```python
from build123d import *

# Parameters (mm, degrees)
F1_DEPTH = 76.2
F3_DEPTH = 59.69


with BuildPart() as f1:
    # F0 (on Front) → F1 (new body)
    with BuildSketch(Plane.XZ):
        Polygon((-9.623217, -31.607002), (0, -26.720898), (9.005067, -12.367957), (23.358002, -30.080097), (23.968766, -5.954943), (42.902432, -17.254066), (29.160259, 4.122653), (48.704684, 14.200249), (23.968766, 14.200249), (31.908695, 39.85231), (12.975028, 16.643301), (12.975028, 45.043796), (5.340484, 18.780973), (0, 43.822274), (-7.790928, 17.559446), (-21.227721, 42.295363), (-13.287797, 13.284104), (-29.167645, 19.086355), (-16.952377, 8.703378), (-36.70152, -2.024551), (-17.56314, -11.757195), (-35.789758, -21.658073), (-9.623217, -15.727157), align=None)
    extrude(amount=F1_DEPTH)

    # F2 (on face) → F3 (cut)
    with BuildSketch(Plane.XZ.offset(76.2)):
        Polygon((21.212701, 12.168249), (26.877798, 30.47086), (10.943028, 10.937917), (10.943028, 30.774279), (5.037519, 10.459334), (-0.322264, 35.591124), (-7.236843, 12.282424), (-14.633635, 25.899247), (-10.289114, 10.025038), (-19.200415, 13.281089), (-13.378382, 8.332362), (-32.335366, -1.965259), (-13.196986, -11.697903), (-21.902551, -16.426851), (-7.591217, -13.18304), (-7.591217, -28.296349), (-1.422014, -25.16399), (8.794351, -8.880393), (21.466165, -24.517956), (22.025383, -2.428849), (36.515134, -11.075958), (26.24216, 4.904228), (40.329954, 12.168249), align=None)
    extrude(amount=-F3_DEPTH, mode=Mode.SUBTRACT)


solid = f1.part
```
The model under review builds one solid part; all positions refer to its coordinate system, in mm. A direction names the side the tool comes from. Give positions to 0.01 mm unless a question says otherwise; leave off trailing zeros. Order: outer loops, then holes, each group sorted by start corner. A loop starts at its lowest first (then second) coordinate and runs counter-clockwise, first axis right, second up. Notation, with made-up numbers: (2.5, 45) - (9.5, 45) arc R12 cw to (9.5, 60) - close; hole circle Ø1 at (-17, 31.25). An arc over 180 degrees is marked (long way). Use CSV: the item, a comma, the result in double quotes. Start each with the question number.
Q1. Tool access review of faces 1 (the flat face through (16, -38, -21)), 2 (the flat face through (36.13, -37.57, -6.72)), 3 (the flat face through (-26.689, -37.567, 3.415)), 4 (the flat face through (22.574, -37.567, 28.41)), 5 (the flat face through (-22.72, -46.77, 3.26)): name each direction out of +Z, -Z, +X, -X, +Y, -Y from which nothing blocks a thin tool from reaching the whole face with its end or side.
Q2. We need section D-D, the plane x = 38.5. Write out the cut boundary in (y, z).
Q3. To check wall thickness, follow line 1 along X through (y, z) = (-13.5, -13.5); line 2 along X through (y, z) = (-5, 37); line 3 along Z through (x, y) = (33.5, -30). State the ranges of each line that lie inside material, in increasing order. Write a range as [from, to].
Q4. The part is to be moulded in two halves that separate along X. For faces 6 (the flat face through (5, 0, -1)), 7 (the flat face through (-14.85, -46.77, -14.83)), 8 (the flat face through (38.796, -37.567, 9.091)), say which applies: +X half, -X half, draft (parallel to the pull), parting line (faces both ways), or undercut.
Q5. We need section C-C, the plane y = -13. Write out the cut boundary in (x, z), and give its area (3 significant figures).
Q6. We need section B-B, the plane x = -25.5. Write out the cut boundary in (y, z), and give its area (3 significant figures).
Q7. We need section A-A, the plane z = -19.5. Write out the cut boundary in (x, y).
Q8. Clearance check with flat-ended pins moving along their axes: pin 1 Ø1.5 at (y, z) = (-62, -15.5) entering from +X; pin 2 Ø2 at (x, z) = (-1, 26.5) entering from +Y; pin 3 Ø8 at (y, z) = (-56.5, -3) entering from -X; pin 4 Ø1.5 at (x, z) = (3, -6) entering from -Y. State where each tip first meets the part, or that it passes through.
Outcome:
1,face 1,"-Z, +Y, -Y"
1,face 2,"+X, +Y, -Y"
1,face 3,"-X, +Y, -Y"
1,face 4,"+Z, +Y, -Y"
1,face 5,"-Y"
2,outline,"(-76.2, -14.63) - (0, -14.63) - (0, -10.41) - (-76.2, -10.41) - close; (-76.2, 8.94) - (0, 8.94) - (0, 14.2) - (-76.2, 14.2) - (-76.2, 12.17) - (-16.51, 12.17) - (-16.51, 11.22) - (-76.2, 11.22) - close"
3,line 1,"x = [-20.77, 8.29], [9.92, 23.78], [36.61, 40.49]"
3,line 2,"x = [-19.78, -18.35], [-2.02, 1.45], [10.64, 12.98], [29.58, 31.03]"
3,line 3,"z = [-11.64, -9.28], [-6.39, -2.63], [6.36, 8.65], [12.17, 14.2]"
4,face 6,"draft"
4,face 7,"undercut"
4,face 8,"+X half"
5,outline,"(-36.7, -2.02) - (-17.56, -11.76) - (-35.79, -21.66) - (-9.62, -15.73) - (-9.62, -31.61) - (0, -26.72) - (9.01, -12.37) - (23.36, -30.08) - (23.97, -5.95) - (42.9, -17.25) - (29.16, 4.12) - (48.7, 14.2) - (23.97, 14.2) - (31.91, 39.85) - (12.98, 16.64) - (12.98, 45.04) - (5.34, 18.78) - (0, 43.82) - (-7.79, 17.56) - (-21.23, 42.3) - (-13.29, 13.28) - (-29.17, 19.09) - (-16.95, 8.7) - close"
5,area,"2,700 mm^2"
6,outline,"(-76.2, -19.33) - (0, -19.33) - (0, -16.07) - (-76.2, -16.07) - close; (-76.2, -7.72) - (0, -7.72) - (0, 4.06) - (-76.2, 4.06) - (-76.2, 1.75) - (-16.51, 1.75) - (-16.51, -5.44) - (-76.2, -5.44) - close; (-76.2, 15.97) - (0, 15.97) - (0, 17.75) - (-76.2, 17.75) - close"
6,area,"852 mm^2"
7,outline,"(-31.82, -76.2) - (-26.27, -76.2) - (-26.27, 0) - (-31.82, 0) - close; (-9.62, -76.2) - (-7.59, -76.2) - (-7.59, -16.51) - (2.13, -16.51) - (2.13, -76.2) - (4.53, -76.2) - (4.53, 0) - (-9.62, 0) - close; (14.78, -76.2) - (17.4, -76.2) - (17.4, -16.51) - (21.59, -16.51) - (21.59, -76.2) - (23.63, -76.2) - (23.63, 0) - (14.78, 0) - close"
8,pin 1,"stops at x = 42.26"
8,pin 2,"stops at y = 0"
8,pin 3,"stops at x = -36.7"
8,pin 4,"stops at y = -16.51"
